Check sheet for the modelled part. Datum: model origin and axes. Units: mm. Give positions to 0.01 mm unless a question says otherwise; leave off trailing zeros. Loops run counter-clockwise (first coordinate to the right, second up) from the corner with the lowest first, then second, coordinate; pieces in that order, holes last.
```python
from build123d import *

# Parameters (mm, degrees)
F1_DEPTH = 127


# Not quite as in the source:
# - ends of sketch curves that miss each other by under 0.0002 mm in the source are joined


with BuildPart() as f1:
    # F0 (on Front) → F1 (new body)
    with BuildSketch(Plane.XZ):
        with BuildLine():
            Line((23.829137, 17.474692), (23.829137, 30.1835566))
            Line((23.829137, 30.1835566), (9.4594934, 30.1835566))
            Line((9.4594934, 30.1835566), (-23.8291116, -7.9430372))
            Line((-23.8291116, -7.9430372), (-23.8291116, -30.1835312))
            Line((-23.8291116, -30.1835312), (-17.474692, -30.1835312))
            ThreePointArc((-17.474692, -30.1835312), (-14.2269141432, -20.357689713), (-4.7658274, -16.1644838))
            Line((-4.7658274, -16.1644838), (-4.7658274, -11.120247))
            ThreePointArc((-4.7658274, -11.120247), (4.2916437043, -5.8802359043), (9.5316594554, 3.1772339438))
            ThreePointArc((9.5316594554, 3.1772339438), (14.8680934033, 12.1382706133), (23.829137, 17.474692))
        make_face()
    extrude(amount=-F1_DEPTH)


solid = f1.part
```
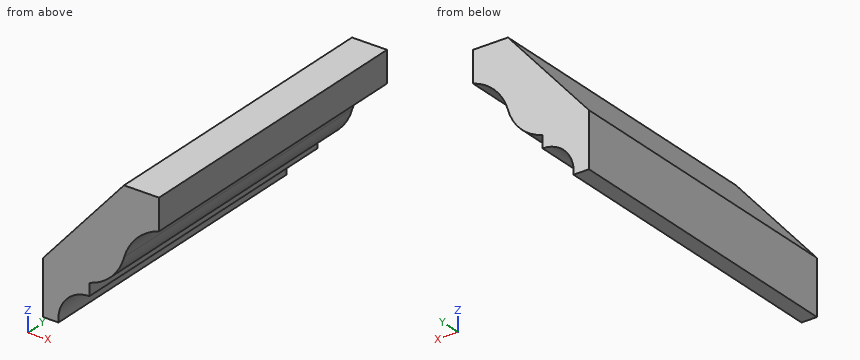
(1) Gauge pin test, flat ends, axial feed: pin 1 Ø3 at (x, y) = (-12, 110) entering from +Z; pin 2 Ø10 at (x, y) = (-16, 17) entering from +Z; pin 3 Ø3 at (x, y) = (12, 72) entering from -Z. Record the tip position at first contact, or that the pin passes through.
(2) Section check A-A on y = 41.5. Record the boundary of the cut face in (x, z).
(3) Material ranges on line 1 (X direction, y = 118, z = -13.5); line 2 (X direction, y = 7.5, z = 28); line 3 (Z direction, x = 21, y = 104.5), recorded low to high.
(4) Section check B-B on x = -3. Record the boundary of the cut face in (y, z).
(5) Section check C-C on z = 8. Record the boundary of the cut face in (x, y), plus the area to 3 significant figures.
Computed values:
1. pin 1: stops at z = 7.32
1. pin 2: stops at z = 6.75
1. pin 3: stops at z = 5.79
2. outline: (-23.83, -30.18) - (-17.47, -30.18) arc R12.77 cw to (-4.77, -16.16) - (-4.77, -11.12) arc R20.28 ccw to (9.53, 3.18) arc R21.22 cw to (23.83, 17.47) - (23.83, 30.18) - (9.46, 30.18) - (-23.83, -7.94) - close
3. line 1: x = -23.83 to -4.77
3. line 2: x = 7.55 to 23.83
3. line 3: z = 16.41 to 30.18
4. outline: (0, -10.56) - (127, -10.56) - (127, 15.91) - (0, 15.91) - close
5. outline: (-9.91, 0) - (11.65, 0) - (11.65, 127) - (-9.91, 127) - close
5. area: 2,740 mm2
